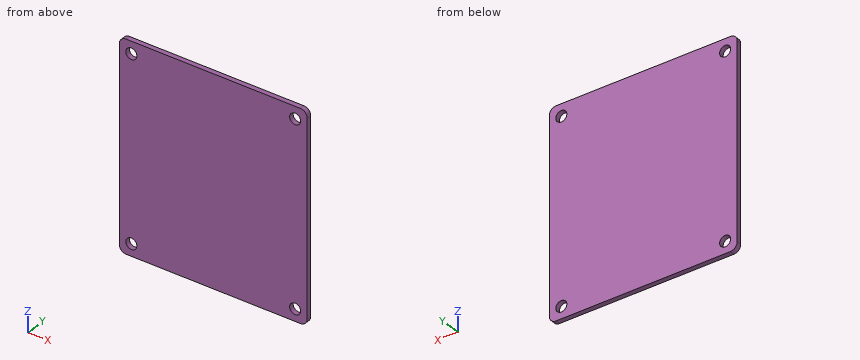
```python
from build123d import *

# Parameters (mm, degrees)
SKETCH1_W           = 54.5
SKETCH1_H           = 60
BOSS_EXTRUDE1_DEPTH = 1.4
SKETCH2_R           = 1.6
CUT_EXTRUDE1_DEPTH  = 2.4
FILLET1_R           = 2


with BuildPart() as part:
    # Sketch1 → Boss-Extrude1 (new body)
    with BuildSketch(Plane(origin=(0, 0, 0), x_dir=(1, 0, 0), z_dir=(0, 1, 0))):
        Rectangle(SKETCH1_W, SKETCH1_H)
    extrude(amount=BOSS_EXTRUDE1_DEPTH)

    # Sketch2 → Cut-Extrude1 (cut, through all)
    with BuildSketch(Plane(origin=(0, 1.4, 0), x_dir=(1, 0, 0), z_dir=(0, 1, 0))):
        with Locations((-23.75, 26.5)):
            Circle(SKETCH2_R)
        with Locations((-23.75, -26.5)):
            Circle(SKETCH2_R)
        with Locations((23.75, -26.5)):
            Circle(SKETCH2_R)
        with Locations((23.75, 26.5)):
            Circle(SKETCH2_R)
    extrude(amount=-CUT_EXTRUDE1_DEPTH, mode=Mode.SUBTRACT)

    # Fillet1
    fillet1_edges = [part.edges().sort_by_distance(p)[0] for p in [
        (-27.25, 0.7, -30),
        (27.25, 0.7, -30),
        (27.25, 0.7, 30),
        (-27.25, 0.7, 30),
    ]]
    fillet(fillet1_edges, radius=FILLET1_R)


solid = part.part
```
Geometry: final body of the model. Coordinates: model frame, mm. Round coordinates to 2 decimals unless told otherwise and drop trailing zeros. Loops run counter-clockwise (first coordinate to the right, second up) from the corner with the lowest first, then second, coordinate; pieces in that order, holes last. Notation, with made-up numbers: (54.5, 88) -> (91.5, 88) arc R32 ccw to (91.5, 126) -> close; hole circle Ø3 at (59.25, 81.5). An arc over 180 degrees is marked (long way). Use one line per item in the form item = value. Start each with the question number.
1) First-contact query: P1, Ø2.5, axis at x = -23.75, z = 26.5, coming from the +Y side. Flat tip, straight axial feed; report the tip coordinate or a pass-through.
2) Section B-B on x = -24. Output: boundary loops of the cut face in (y, z).
3) Section A-A on z = -26.5. Output: boundary loops of the cut face in (x, y), then the cut area to 3 significant figures.
4) Line query: L1, parallel to X at y = 1.1, z = 26.5; L2, parallel to Z at x = -23.75, y = 0.85. Output: solid intervals per line, ascending.
Response:
q1.P1 = through
q2.outline = (0, -30) -> (1.4, -30) -> (1.4, -28.08) -> (0, -28.08) -> close; (0, -24.92) -> (1.4, -24.92) -> (1.4, 24.92) -> (0, 24.92) -> close; (0, 28.08) -> (1.4, 28.08) -> (1.4, 30) -> (0, 30) -> close
q3.outline = (-27.25, 0) -> (-25.35, 0) -> (-25.35, 1.4) -> (-27.25, 1.4) -> close; (-22.15, 0) -> (22.15, 0) -> (22.15, 1.4) -> (-22.15, 1.4) -> close; (25.35, 0) -> (27.25, 0) -> (27.25, 1.4) -> (25.35, 1.4) -> close
q3.area = 67.3 mm^2
q4.L1 = -27.25 to -25.35, -22.15 to 22.15, 25.35 to 27.25
q4.L2 = -30 to -28.1, -24.9 to 24.9, 28.1 to 30
